from build123d import *

# Parameters (mm, degrees)
F0_R     = 47.037606
F1_DEPTH = 980
F2_R     = 25.753318
F3_DEPTH = 25
F5_DEPTH = 25


with BuildPart() as f1:
    # F0 (on Front) → F1 (new body)
    with BuildSketch(Plane.XZ):
        Circle(F0_R)
    extrude(amount=F1_DEPTH)

    # F2 (on Front) → F3 (join)
    with BuildSketch(Plane.XZ):
        Circle(F2_R)
    extrude(amount=F3_DEPTH)

    # F4 (on Top) → F5 (cut)
    with BuildSketch(Plane.XY):
        with BuildLine():
            add(Edge.make_bspline(
                [(0, 70.394285), (-52.129742, 70.394285), (-26.064871, -35.197143), (0, -140.78857), (26.064871, -35.197143), (52.129742, 70.394285), (0, 70.394285)],
                knots=[0, 0, 0, 2.094395, 2.094395, 4.18879, 4.18879, 6.283185, 6.283185, 6.283185], degree=2, weights=[1, 0.5, 1, 0.5, 1, 0.5, 1]))
        make_face()
    extrude(amount=-F5_DEPTH, mode=Mode.SUBTRACT)


solid = f1.part
Geometry: final body of the model. Coordinates: model frame, mm. A direction names the side the tool comes from. Give positions to 0.01 mm unless a question says otherwise; leave off trailing zeros. Loops run counter-clockwise (first coordinate to the right, second up) from the corner with the lowest first, then second, coordinate; pieces in that order, holes last. Notation, with made-up numbers: M 57.5,35 L 96.5,35 A15 cw 96.5,49 Z; hole C 88,-11.75 d5. An arc over 180 degrees is marked long. Put each result on its own line as item: value.
1) Reachability of faces 4 (the flat face through (-1, -980, 1)), 5 (the flat face through (0, -22, 0)) from +Z, -Z, +X, -X, +Y, -Y: full face, straight path, thin tool, end or side. Return the list, or none.
Computed values:
face 4: +Z, -Z, +X, -X, -Y
face 5: +Y
2) Mould query, pull axis X, two halves, no side actions, for faces 1 (the flat face through (-1, 0, 1)), 2 (the cylindrical face through (25.29, -483.14, 39.66)), 3 (the flat face through (0, -22, -25)). Classes: released by +X, released by -X, zero draft, split by the parting line, or undercut.
Computed values:
face 1: zero draft
face 2: split by the parting line
face 3: undercut
3) Cut plane A-A, the plane y = -446.5. Return the cut outline in (x, z).
Computed values:
outline: C 0,0 d94.08
4) First-contact query: P1, Ø5, axis at x = -6, y = -813, coming from the +Z side; P2, Ø10, axis at x = -29, y = -513.5, coming from the -Z side; P3, Ø2, axis at y = -260.5, z = 3.5, coming from the +X side. Flat tips, straight axial feed; report the tip coordinate or a pass-through.
Computed values:
P1: stops at z = 46.91
P2: stops at z = -40.45
P3: stops at x = 46.97
5) Material intervals for L1, parallel to Z at x = 1, y = -71; L2, parallel to X at y = -427.5, z = 2; L3, parallel to Z at x = -22.5, y = -203, sorted ascending. Write a range as from..to.
Computed values:
L1: z = -47.03..47.03
L2: x = -47..47
L3: z = -41.31..41.31
6) Cut plane B-B, the plane z = 27.5. Return the cut outline in (x, y), plus the area to 3 significant figures.
Computed values:
outline: M -38.16,-980 L 38.16,-980 L 38.16,0 L -38.16,0 Z
area: 74,800 mm^2
